Source: CAD feature listing. Evaluate the final solid. Frame: model axes, mm. Round coordinates to 2 decimals unless told otherwise and drop trailing zeros. Write each loop counter-clockwise with the first axis right and the second up, starting at its lowest first coordinate (ties: lowest second). Pieces come first, ordered by that corner, then holes. Notation, with made-up numbers: M 37,49.5 L 95,49.5 A35 ccw 95,81.5 Z; hole C 66,-16 d11. An arc over 180 degrees is marked long. Use a Markdown table: item, result.
Autodesk Inventor part; units mm, degrees
ref_plane "YZ Plane" through (0, 0, 0) normal (1, 0, 0) x (0, 1, 0)
ref_plane "XZ Plane" through (0, 0, 0) normal (0, 1, 0) x (-1, 0, 0)
ref_plane "XY Plane" through (0, 0, 0) normal (0, 0, 1) x (1, 0, 0)
sketch "Sketch2" plane through (0, 0, 0) normal (0, 1, 0) x (-1, 0, 0)
  line L0 (0, 0) -> (125.1, 0)
  line L1 (125.1, 0) -> (125.1, -70.1)
  line L2 (125.1, -70.1) -> (0, -70.1)
  line L3 (0, -70.1) -> (0, 0)
  dimension "d5" = 70.1
  dimension "d6" = 125.1
extrude "Extrusion2" add sketch "Sketch2" along normal blind 4
fillet "Fillet1" radius 2 4 edges at (-125.1, 2, 0) (-125.1, 2, -70.1) (0, 2, 0) (0, 2, -70.1)
sketch "Sketch4" plane through (0, 0, 0) normal (0, -1, 0) x (1, 0, 0)
  line L0 (-60.7951, -25.715) -> (-60.7951, -33.115)
  line L1 (-60.7951, -33.115) -> (-70.9551, -33.115)
  line L2 (-70.9551, -25.715) -> (-70.9551, -33.115)
  line L3 (-60.7951, -25.715) -> (-70.9551, -25.715)
  line L4 (-70.2151, -31.515) -> (-66.6151, -31.515)
  line L5 (-66.6151, -31.515) -> (-66.6151, -26.315)
  line L6 (-66.6151, -26.315) -> (-70.2151, -26.315)
  line L7 (-70.2151, -26.315) -> (-70.2151, -31.515)
  line L8 (-65.1351, -31.515) -> (-61.5351, -31.515)
  line L9 (-61.5351, -31.515) -> (-61.5351, -26.315)
  line L10 (-61.5351, -26.315) -> (-65.1351, -26.315)
  line L11 (-65.1351, -26.315) -> (-65.1351, -31.515)
  line L12 (-87.4551, -25.715) -> (-87.4551, -33.115)
  line L13 (-87.4551, -33.115) -> (-97.6151, -33.115)
  line L14 (-97.6151, -25.715) -> (-97.6151, -33.115)
  line L15 (-87.4551, -25.715) -> (-97.6151, -25.715)
  line L16 (-96.8751, -31.515) -> (-93.2751, -31.515)
  line L17 (-93.2751, -31.515) -> (-93.2751, -26.315)
  line L18 (-93.2751, -26.315) -> (-96.8751, -26.315)
  line L19 (-96.8751, -26.315) -> (-96.8751, -31.515)
  line L20 (-91.7951, -31.515) -> (-88.1951, -31.515)
  line L21 (-88.1951, -31.515) -> (-88.1951, -26.315)
  line L22 (-88.1951, -26.315) -> (-91.7951, -26.315)
  line L23 (-91.7951, -26.315) -> (-91.7951, -31.515)
  line L24 (-26.0551, -25.715) -> (-26.0551, -33.115)
  line L25 (-26.0551, -33.115) -> (-36.2151, -33.115)
  line L26 (-36.2151, -25.715) -> (-36.2151, -33.115)
  line L27 (-26.0551, -25.715) -> (-36.2151, -25.715)
  line L28 (-35.4751, -31.515) -> (-31.8751, -31.515)
  line L29 (-31.8751, -31.515) -> (-31.8751, -26.315)
  line L30 (-31.8751, -26.315) -> (-35.4751, -26.315)
  line L31 (-35.4751, -26.315) -> (-35.4751, -31.515)
  line L32 (-30.3951, -31.515) -> (-26.7951, -31.515)
  line L33 (-26.7951, -31.515) -> (-26.7951, -26.315)
  line L34 (-26.7951, -26.315) -> (-30.3951, -26.315)
  line L35 (-30.3951, -26.315) -> (-30.3951, -31.515)
  line L36 (-101.8351, -28.915) -> (-21.8351, -28.915) construction
  line L37 (-97.6351, -33.115) -> (-26.0351, -33.115) construction
  line L38 (-26.0351, -24.715) -> (-97.6351, -24.715) construction
  arc A0 (-97.6351, -24.715) -> (-97.6351, -33.115) centre (-97.6351, -28.915) ccw
  arc A1 (-26.0351, -33.115) -> (-26.0351, -24.715) centre (-26.0351, -28.915) ccw
  line L39 (-97.6151, -25.715) -> (-97.6151, -10.355) construction
  line L40 (-26.0551, -25.715) -> (-26.0551, -14.2023) construction
  line L41 (-101.8351, -28.915) -> (-101.8351, -10.355) construction
  line L42 (-101.8351, -10.355) -> (-97.6151, -10.355) construction
  line L43 (-26.0551, -14.2023) -> (-21.8351, -14.2023) construction
  line L44 (-21.8351, -14.2023) -> (-21.8351, -28.915) construction
  line L45 (-101.8351, -28.915) -> (-83.2351, -28.915) construction
  line L46 (-97.6351, -33.115) -> (-87.4351, -33.115)
  line L47 (-87.4351, -24.715) -> (-97.6351, -24.715)
  arc A2 (-97.6351, -24.715) -> (-97.6351, -33.115) centre (-97.6351, -28.915) ccw
  arc A3 (-87.4351, -33.115) -> (-87.4351, -24.715) centre (-87.4351, -28.915) ccw
  line L48 (-75.1751, -28.915) -> (-56.5751, -28.915) construction
  line L49 (-70.9751, -33.115) -> (-60.7751, -33.115)
  line L50 (-60.7751, -24.715) -> (-70.9751, -24.715)
  arc A4 (-70.9751, -24.715) -> (-70.9751, -33.115) centre (-70.9751, -28.915) ccw
  arc A5 (-60.7751, -33.115) -> (-60.7751, -24.715) centre (-60.7751, -28.915) ccw
  line L51 (-40.4351, -28.915) -> (-21.8351, -28.915) construction
  line L52 (-36.2351, -33.115) -> (-26.0351, -33.115)
  line L53 (-26.0351, -24.715) -> (-36.2351, -24.715)
  arc A6 (-36.2351, -24.715) -> (-36.2351, -33.115) centre (-36.2351, -28.915) ccw
  arc A7 (-26.0351, -33.115) -> (-26.0351, -24.715) centre (-26.0351, -28.915) ccw
  point P0 (0, 0)
  point P1 (-61.8351, -28.915)
  point P2 (-92.5351, -28.915)
  point P3 (-65.8751, -28.915)
  point P4 (-31.1351, -28.915)
  point P5 (-97.6351, -24.715)
  point P6 (-26.0351, -33.115)
  point P7 (-26.0351, -24.715)
  dimension "d10" = 80
  dimension "d11" = 0
  dimension "d12" = 1
  dimension "d13" = 4.22
  dimension "d14" = 4.22
  dimension "d15" = 4.22
  dimension "d16" = 4.22
  dimension "d17" = 4.22
extrude "Extrusion3" cut sketch "Sketch4" against normal blind 10 contours L3 L2 L49 A4 L50 A5 L0 | L0 L1 L2 L3 | L7 L6 L5 L4 | L11 L10 L9 L8 | L15 L14 L46 A0 L47 A3 L12 | L12 L13 L14 L15 | L19 L18 L17 L16 | L23 L22 L21 L20 | L27 L26 L52 A6 L53 A1 L24 | L24 L25 L26 L27 | L31 L30 L29 L28 | L35 L34 L33 L32
sketch "Sketch5" plane through (0, 4, 0) normal (0, 1, 0) x (1, 0, 0)
  line L0 (-44.9757, 55.92) -> (-50.6457, 55.92) construction
  arc A0 (-50.6457, 55.92) -> (-50.7457, 55.82) centre (-50.6457, 55.82) ccw construction
  line L1 (-50.7457, 55.82) -> (-50.7457, 55.006) construction
  arc A1 (-51.0707, 54.4431) -> (-50.7457, 55.006) centre (-51.3957, 55.006) ccw construction
  line L2 (-51.0707, 54.4431) -> (-51.2107, 54.3623) construction
  arc A2 (-51.2107, 54.3623) -> (-51.2607, 54.2757) centre (-51.1607, 54.2757) ccw construction
  line L3 (-51.2607, 54.2757) -> (-51.2607, 52.82) construction
  line L4 (-51.2607, 52.82) -> (-44.3607, 52.82) construction
  line L5 (-44.3607, 52.82) -> (-44.3607, 54.2757) construction
  arc A3 (-44.3607, 54.2757) -> (-44.4107, 54.3623) centre (-44.4607, 54.2757) ccw construction
  line L6 (-44.4107, 54.3623) -> (-44.5507, 54.4431) construction
  arc A4 (-44.8757, 55.006) -> (-44.5507, 54.4431) centre (-44.2257, 55.006) ccw construction
  line L7 (-44.8757, 55.006) -> (-44.8757, 55.82) construction
  arc A5 (-44.8757, 55.82) -> (-44.9757, 55.92) centre (-44.9757, 55.82) ccw construction
  line L8 (-50.8957, 56.32) -> (-44.7257, 56.32) construction
  arc A6 (-44.4757, 56.07) -> (-44.7257, 56.32) centre (-44.7257, 56.07) ccw construction
  line L9 (-44.4757, 56.07) -> (-44.4757, 55.006) construction
  arc A7 (-44.4757, 55.006) -> (-44.3507, 54.7895) centre (-44.2257, 55.006) ccw construction
  line L10 (-44.3507, 54.7895) -> (-44.0857, 54.6365) construction
  arc A8 (-43.9607, 54.42) -> (-44.0857, 54.6365) centre (-44.2107, 54.42) ccw construction
  line L11 (-43.9607, 54.42) -> (-43.9607, 52.82) construction
  arc A9 (-44.3607, 52.42) -> (-43.9607, 52.82) centre (-44.3607, 52.82) ccw construction
  line L12 (-44.3607, 52.42) -> (-51.2607, 52.42) construction
  arc A10 (-51.6607, 52.82) -> (-51.2607, 52.42) centre (-51.2607, 52.82) ccw construction
  line L13 (-51.6607, 52.82) -> (-51.6607, 54.42) construction
  arc A11 (-51.5357, 54.6365) -> (-51.6607, 54.42) centre (-51.4107, 54.42) ccw construction
  line L14 (-51.5357, 54.6365) -> (-51.2707, 54.7895) construction
  arc A12 (-51.2707, 54.7895) -> (-51.1457, 55.006) centre (-51.3957, 55.006) ccw construction
  line L15 (-51.1457, 55.006) -> (-51.1457, 56.07) construction
  arc A13 (-50.8957, 56.32) -> (-51.1457, 56.07) centre (-50.8957, 56.07) ccw construction
  line L16 (-23, 54.87) -> (-102.1, 54.87) construction
  line L17 (-29.45, 61.32) -> (-95.65, 61.32)
  line L18 (-95.65, 48.42) -> (-29.45, 48.42)
  arc A14 (-29.45, 48.42) -> (-29.45, 61.32) centre (-29.45, 54.87) ccw
  arc A15 (-95.65, 61.32) -> (-95.65, 48.42) centre (-95.65, 54.87) ccw
  line L19 (0, 2) -> (0, 68.1)
  line L20 (-125.1, 68.1) -> (-125.1, 2)
  point P0 (0, 0)
  point P1 (-62.55, 54.87)
  dimension "d20" = 23
  dimension "d21" = 5
  dimension "d22" = 4
  dimension "d23" = 23
extrude "Extrusion4" cut sketch "Sketch5" against normal blind 7.75
equation "\"d14\" = d13"
equation "\"d15\" = d14"
equation "\"d16\" = d15"
equation "\"d17\" = d16"
equation "\"d23\" = d20"
equation "\"BendRadius\" = Thickness"
equation "\"BendReliefWidth\" = Thickness"
equation "\"BendReliefDepth\" = 0.5 * Thickness"
equation "\"CornerReliefSize\" = 4 * Thickness"
equation "\"MinimumRemnant\" = 2 * Thickness"
equation "\"TransitionRadius\" = BendRadius"
equation "\"JacobiRadiusSize\" = Thickness"
equation "\"GapSize\" = Thickness"
properties part number "back"
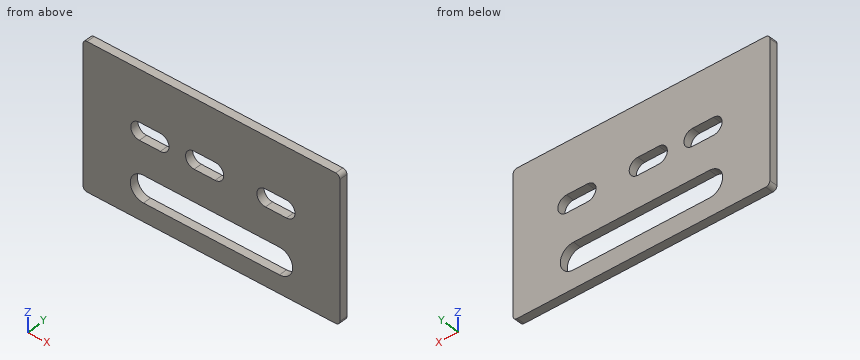
Q1. Line query: L1, parallel to Z at x = -95, y = 0.6 (3 decimals); L2, parallel to X at y = 3.7, z = -29; L3, parallel to Z at x = -86, y = 3.5. Output: solid intervals per line, ascending.
Results are:
| item | result |
|---|---|
| L1 | -70.1 to -61.32, -48.42 to -33.115, -24.715 to 0 |
| L2 | -125.1 to -101.83, -83.24 to -75.17, -56.58 to -40.43, -21.84 to 0 |
| L3 | -70.1 to -61.32, -48.42 to -32.86, -24.97 to 0 |
Q2. Section A-A on x = -91.5. Return loops of the section in (y, z) (3 decimals), plus the area to 3 significant figures.
Results are:
| item | result |
|---|---|
| outline | M 0,-70.1 L 4,-70.1 L 4,-61.32 L 0,-61.32 Z; M 0,-48.42 L 4,-48.42 L 4,-33.115 L 0,-33.115 Z; M 0,-24.715 L 4,-24.715 L 4,0 L 0,0 Z |
| area | 195 mm^2 |
Q3. Section B-B on y = 2.7. Return loops of the section in (x, z) (3 decimals), plus the area to 3 significant figures.
Results are:
| item | result |
|---|---|
| outline | M -125.1,-68.1 A2 ccw -123.1,-70.1 L -2,-70.1 A2 ccw 0,-68.1 L 0,-2 A2 ccw -2,0 L -123.1,0 A2 ccw -125.1,-2 Z; hole M -97.635,-33.115 L -87.435,-33.115 A4.2 ccw -87.435,-24.715 L -97.635,-24.715 A4.2 ccw Z; hole M -95.65,-61.32 L -29.45,-61.32 A6.45 ccw -29.45,-48.42 L -95.65,-48.42 A6.45 ccw Z; hole M -70.975,-33.115 L -60.775,-33.115 A4.2 ccw -60.775,-24.715 L -70.975,-24.715 A4.2 ccw Z; hole M -36.235,-33.115 L -26.035,-33.115 A4.2 ccw -26.035,-24.715 L -36.235,-24.715 A4.2 ccw Z |
| area | 7,360 mm^2 |
Q4. Section C-C on z = -54.87. Return loops of the section in (x, y), plus the area to 3 significant figures.
Results are:
| item | result |
|---|---|
| outline | M -125.1,0 L -102.1,0 L -102.1,4 L -125.1,4 Z; M -23,0 L 0,0 L 0,4 L -23,4 Z |
| area | 184 mm^2 |
